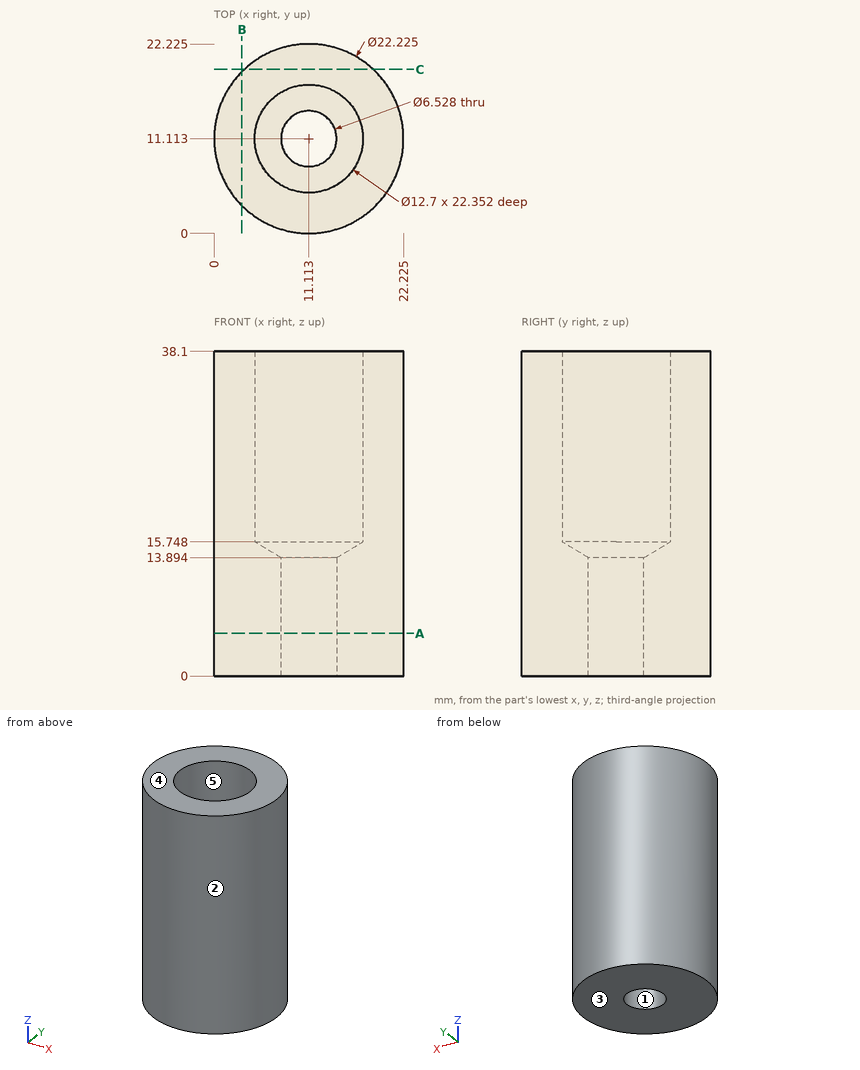
Part print with two shaded views. Sizes in mm from the minimum x, y, z corner. A direction names the side the tool comes from. Round coordinates to 2 decimals unless told otherwise and drop trailing zeros. Loops run counter-clockwise (first coordinate to the right, second up) from the corner with the lowest first, then second, coordinate; pieces in that order, holes last.
Item 1: Drill centre lines: line 1 along Y through (x, z) = (11.25, 18.5) (1 decimal); line 2 along Y through (x, z) = (9.25, 2.5) (1 decimal); line 3 along X through (y, z) = (17, 19) (1 decimal). Where is each one in solid material? Low to high.
Item 2: Saw through at A-A (z = 5). List the corners of the cut face in (x, y) (1 decimal).
Item 3: Which spindle directions (+Z, -Z, +X, -X, +Y, -Y) get a long thin tool onto all of the face, cutting with end or side? Do the marked faces 4 and 5. Say none if no direction does.
Item 4: Saw through at C-C (y = 19.25). List the corners of the cut face in (x, z) (1 decimal), then the cut area to 3 significant figures.
Item 5: Two-plate mould, pull along X, no slides. Class the marked faces 1, 2 and 3: released by +X, released by -X, zero draft, split by the parting line, or undercut.
Item 6: Saw through at B-B (x = 3.25). List the corners of the cut face in (y, z) (1 decimal).
Item 7: Pin check, flat tips, straight feed: P1, Ø11.5, axis at x = 11.11, y = 11.11, coming from the +Z side; P2, Ø1, axis at x = 4.5, z = 5, coming from the -Y side; P3, Ø6, axis at x = 2.5, z = 17, coming from the -Y side. Stop position of each tip, or through.
Worked answers:
1. line 1: y = 0 to 4.8, 17.5 to 22.2
1. line 2: y = 0.2 to 8.4, 13.8 to 22.1
1. line 3: x = 1.7 to 8.7, 13.5 to 20.5
2. outline: circle Ø22.2 at (11.1, 11.1); hole circle Ø6.5 at (11.1, 11.1)
3. face 4: +Z, +X, -X, +Y, -Y
3. face 5: +Z
4. outline: (3.5, 0) - (18.7, 0) - (18.7, 38.1) - (3.5, 38.1) - close
4. area: 577 mm2
5. face 1: undercut
5. face 2: split by the parting line
5. face 3: zero draft
6. outline: (3.3, 0) - (19, 0) - (19, 38.1) - (3.3, 38.1) - close
7. P1: stops at z = 15.39
7. P2: stops at y = 1.83
7. P3: stops at y = 1.52
